Autodesk Inventor part; units mm, degrees
ref_plane "YZ Plane" through (0, 0, 0) normal (1, 0, 0) x (0, 1, 0)
ref_plane "XZ Plane" through (0, 0, 0) normal (0, 1, 0) x (-1, 0, 0)
ref_plane "XY Plane" through (0, 0, 0) normal (0, 0, 1) x (1, 0, 0)
sketch "Boceto1" plane through (0, 0, 0) normal (0, 0, 1) x (1, 0, 0)
  circle A0 centre (0, 0) radius 8.9
  line L0 (6.2933, -6.2933) -> (-6.2933, -6.2933)
  line L1 (-6.2933, -6.2933) -> (-6.2933, 6.2933)
  line L2 (-6.2933, 6.2933) -> (6.2933, 6.2933)
  line L3 (6.2933, 6.2933) -> (6.2933, -6.2933)
  dimension "d0" = 17.8
  dimension "d1" = 12.5865
  dimension "d2" = 12.5865
extrude "Extrusión1" add sketch "Boceto1" along normal blind 32 contours L3 L0 L1 L2
sketch "Boceto2" plane through (0, 0, 0) normal (0, 1, 0) x (-1, 0, 0)
  line L0 (6.2933, 0) -> (-6.2933, 0)
  line L1 (-6.2933, 0) -> (-6.2933, 2)
  line L2 (-6.2933, 2) -> (6.2933, 2)
  line L3 (6.2933, 2) -> (6.2933, 0)
  line L4 (6.2933, 5) -> (-6.2933, 5)
  line L5 (-6.2933, 5) -> (-6.2933, 7)
  line L6 (-6.2933, 7) -> (6.2933, 7)
  line L7 (6.2933, 7) -> (6.2933, 5)
  line L8 (6.2933, 10) -> (-6.2933, 10)
  line L9 (-6.2933, 10) -> (-6.2933, 12)
  line L10 (-6.2933, 12) -> (6.2933, 12)
  line L11 (6.2933, 12) -> (6.2933, 10)
  line L12 (6.2933, 15) -> (-6.2933, 15)
  line L13 (-6.2933, 15) -> (-6.2933, 17)
  line L14 (-6.2933, 17) -> (6.2933, 17)
  line L15 (6.2933, 17) -> (6.2933, 15)
  line L16 (6.2933, 20) -> (-6.2933, 20)
  line L17 (-6.2933, 20) -> (-6.2933, 22)
  line L18 (-6.2933, 22) -> (6.2933, 22)
  line L19 (6.2933, 22) -> (6.2933, 20)
  line L20 (6.2933, 25) -> (-6.2933, 25)
  line L21 (-6.2933, 25) -> (-6.2933, 27)
  line L22 (-6.2933, 27) -> (6.2933, 27)
  line L23 (6.2933, 27) -> (6.2933, 25)
  line L24 (6.2933, 30) -> (-6.2933, 30)
  line L25 (-6.2933, 30) -> (-6.2933, 32)
  line L26 (-6.2933, 32) -> (6.2933, 32)
  line L27 (6.2933, 32) -> (6.2933, 30)
  line L28 (-6.2933, 0) -> (6.2933, 0)
  line L29 (-6.2933, 0) -> (6.2933, 5)
  line L30 (-6.2933, 1.883) -> (6.2933, 6.883)
  line L31 (-6.2933, 6.883) -> (6.2933, 11.883)
  line L32 (-6.2933, 5) -> (6.2933, 10)
  line L33 (-6.2933, 11.883) -> (6.2933, 16.883)
  line L34 (-6.2933, 10) -> (6.2933, 15)
  line L35 (-6.2933, 16.883) -> (6.2933, 21.883)
  line L36 (-6.2933, 15) -> (6.2933, 20)
  line L37 (-6.2933, 21.883) -> (6.2933, 26.883)
  line L38 (-6.2933, 20) -> (6.2933, 25)
  line L39 (-6.2933, 26.883) -> (6.2933, 31.883)
  line L40 (-6.2933, 25) -> (6.2933, 30)
  line L41 (6.2933, 0) -> (4.2933, 0)
  line L42 (4.2933, 0) -> (4.2933, 7)
  line L43 (4.2933, 7) -> (6.2933, 7)
  line L44 (6.2933, 7) -> (6.2933, 0)
  line L45 (-6.2933, 0) -> (-4.2933, 0)
  line L46 (-4.2933, 0) -> (-4.2933, 7)
  line L47 (-4.2933, 7) -> (-6.2933, 7)
  line L48 (-6.2933, 7) -> (-6.2933, 0)
  point P0 (0, 0)
  point P1 (0, 5)
  point P2 (0, 10)
  point P3 (0, 15)
  point P4 (0, 20)
  point P5 (0, 25)
  point P6 (0, 30)
  point P7 (1.5531, 30)
  point P8 (-5.9988, 27)
  point P9 (1.5531, 25)
  point P10 (-5.9988, 22)
  point P11 (1.5531, 20)
  point P12 (-5.9988, 17)
  point P13 (1.5531, 15)
  point P14 (-5.9988, 12)
  point P15 (1.5531, 10)
  point P16 (-5.9988, 7)
  point P17 (1.5531, 5)
  point P18 (-5.9988, 2)
  point P19 (-1.2586, 2)
  point P20 (-1.2587, 7)
  point P21 (-1.2587, 12)
  point P22 (-1.2587, 17)
  point P23 (-1.2586, 22)
  point P24 (-1.2586, 27)
  point P25 (4.2933, 5)
  point P26 (4.2933, 2)
  point P27 (-4.2933, 2)
  point P28 (-4.2933, 5)
  dimension "d5" = 2
  dimension "d8" = 5
  dimension "d13" = 1.75
  dimension "d16" = 5
  dimension "d23" = 2
  dimension "d24" = 2
extrude "Extrusión2" cut sketch "Boceto2" against normal mid plane 30 contours L0 L42 L2 L3 | L0 L46 L29 L2 L42 | L2 L42 L29 L44 | L0 L29 L46 | L29 L42 L4 | L4 L42 L30 L7 | L1 L30 L2 L46 L29 | L46 L2 L29 | L4 L30 L42 | L30 L42 L6 L7 | L1 L2 L30 | L2 L30 L46 | L4 L46 L32 L6 L42 L30 | L48 L4 L46 L30 L2 | L4 L32 L46 | L5 L31 L6 L46 L32 | L46 L6 L32 | L6 L31 L8 L32 | L5 L6 L31 | L8 L31 L11 | L8 L34 L10 L11 L31 | L9 L33 L10 L34 | L9 L10 L33 | L10 L33 L12 L34 | L12 L33 L15 | L12 L36 L14 L15 L33 | L13 L35 L14 L36 | L13 L14 L35 | L14 L35 L16 L36 | L16 L35 L19 | L16 L38 L18 L19 L35 | L17 L37 L18 L38 | L17 L18 L37 | L18 L37 L20 L38 | L20 L37 L23 | L20 L40 L22 L23 L37 | L21 L39 L22 L40 | L21 L22 L39 | L22 L39 L24 L40 | L24 L39 L27 | L24 L25 L26 L27 L39 keep common part
sketch "Boceto3" plane through (0, 0, 0) normal (0, 0, -1) x (-1, 0, 0)
  circle A0 centre (0, 0) radius 2
  dimension "d25" = 4
extrude "Extrusión3" cut sketch "Boceto3" against normal blind 20
properties part number "_3DPrint"
Can you work these out from the model? Positions are in its coordinate system, mm. A direction names the side the tool comes from. Coordinates: 2 decimals unless noted, no trailing zeros. Order: outer loops, then holes, each group sorted by start corner. A loop starts at its lowest first (then second) coordinate and runs counter-clockwise, first axis right, second up.
1. For faces 1 (the face through (-4.293, 0, 3)), 2 (the face through (2, 0, 30)), 3 (the face through (6.293, 0, 31)), which set-ups out of +Z, -Z, +X, -X, +Y, -Y let a thin tool reach every point of the face, with its end or its side?
2. If we section it at A-A (x = 5): Please give me the cut outline in (y, z).
3. Thinking about a two-plate mould opening in Z: for faces 4 (the face through (2.276, 0.088, 28.479)), 5 (the face through (0, 0, 32)), 6 (the face through (-6.293, 0, 26)), which applies, +Z half, -Z half, draft (parallel to the pull), parting line (faces both ways), or undercut?
4. If we section it at B-B (x = -3): Please give me the cut outline in (y, z), then the cut area to 3 significant figures.
5. If we section it at D-D (z = 17.5): Please give me the cut outline in (x, y), then the cut area to 3 significant figures.
6. If we section it at C-C (y = 0): Give the number of separate pieces and of enclosed holes in the cut face, then the cut area to 3 significant figures.
7. I need wall thicknesses on line 1 (Y direction, x = 0, z = 1.1); line 2 (X direction, y = -0.25, z = 3.5). Which ranges of each line are inside material? Lowest first, please.
Entries:
1. face 1: +Y, -Y
1. face 2: +X, +Y, -Y
1. face 3: +Z, -Z, +X, +Y, -Y
2. outline: (-6.29, 0) - (6.29, 0) - (6.29, 7.4) - (-6.29, 7.4) - close; (-6.29, 10) - (6.29, 10) - (6.29, 12.4) - (-6.29, 12.4) - close; (-6.29, 15) - (6.29, 15) - (6.29, 17.4) - (-6.29, 17.4) - close; (-6.29, 20) - (6.29, 20) - (6.29, 22.4) - (-6.29, 22.4) - close; (-6.29, 25) - (6.29, 25) - (6.29, 27.4) - (-6.29, 27.4) - close; (-6.29, 30) - (6.29, 30) - (6.29, 32) - (-6.29, 32) - close
3. face 4: undercut
3. face 5: +Z half
3. face 6: draft
4. outline: (-6.29, 0) - (6.29, 0) - (6.29, 2) - (-6.29, 2) - close; (-6.29, 5) - (6.29, 5) - (6.29, 7) - (-6.29, 7) - close; (-6.29, 8.69) - (6.29, 8.69) - (6.29, 12) - (-6.29, 12) - close; (-6.29, 13.69) - (6.29, 13.69) - (6.29, 17) - (-6.29, 17) - close; (-6.29, 18.69) - (6.29, 18.69) - (6.29, 22) - (-6.29, 22) - close; (-6.29, 23.69) - (6.29, 23.69) - (6.29, 27) - (-6.29, 27) - close; (-6.29, 28.69) - (6.29, 28.69) - (6.29, 32) - (-6.29, 32) - close
4. area: 259 mm2
5. outline: (0, -6.29) - (4.74, -6.29) - (4.74, 6.29) - (0, 6.29) - (0, 2) arc R2 cw to (0, -2) - close
5. area: 53.4 mm2
6. separate pieces: 7
6. enclosed holes: 0
6. area: 205 mm2
7. line 1: y = -6.29 to -2, 2 to 6.29
7. line 2: x = -6.29 to -4.29, 4.29 to 6.29
